The listing builds one solid part. Answer for the finished solid, in the listing's coordinates (mm). Face numbers are marked on the shaded views. A direction names the side the tool comes from. Round coordinates to 2 decimals unless told otherwise and drop trailing zeros. Write each loop counter-clockwise with the first axis right and the second up, starting at its lowest first coordinate (ties: lowest second). Pieces come first, ordered by that corner, then holes. Notation, with made-up numbers: (57, 32) - (108, 32) arc R20 cw to (108, 65) - close; hole circle Ø5 at (69.5, -26.5). An arc over 180 degrees is marked (long way). Return JSON: item names as keys, results as strings. Group by question number.
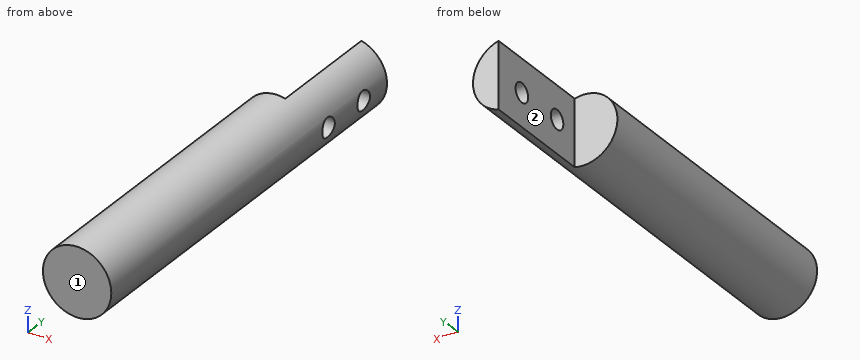
from build123d import *

# Parameters (mm, degrees)
SKETCH_1_R          = 3.175
EXTRUDE_1_DEPTH     = 57.15
CUT_EXTRUDE_1_DEPTH = 10.795
SKETCH_3_R          = 0.889
CUT_EXTRUDE_2_DEPTH = 10.795
SKETCH_4_W          = 3.926157487
SKETCH_4_H          = 0.79375
CUT_EXTRUDE_3_DEPTH = 8.573
SKETCH_5_R          = 3.774888962
CUT_EXTRUDE_4_DEPTH = 18


with BuildPart() as part:
    # 草图1 → 凸台-拉伸1 (new body)
    with BuildSketch(Plane(origin=(0, 0, 0), x_dir=(1, 0, 0), z_dir=(0, 1, 0))):
        Circle(SKETCH_1_R)
    extrude(amount=EXTRUDE_1_DEPTH)

    # 草图2 → 切除-拉伸1 (cut)
    with BuildSketch(Plane(origin=(0, 57.15, 0), x_dir=(1, 0, 0), z_dir=(0, 1, 0))):
        Polygon((-0.794, 3.175), (0.794, 3.175), (0.794, -3.175), (-3.175, -3.175), (-3.175, 3.175), align=None)
    extrude(amount=-CUT_EXTRUDE_1_DEPTH, mode=Mode.SUBTRACT)

    # 草图3 → 切除-拉伸2 (cut)
    with BuildSketch(Plane.ZY.offset(-0.794)):
        with Locations((0, 53.855)):
            Circle(SKETCH_3_R)
        with Locations((0, 48.855)):
            Circle(SKETCH_3_R)
    extrude(amount=-CUT_EXTRUDE_2_DEPTH, mode=Mode.SUBTRACT)

    # 草图4 → 切除-拉伸3 (cut)
    with BuildSketch(Plane.XZ):
        with Locations((-0.018009896, -2.778125)):
            Rectangle(SKETCH_4_W, SKETCH_4_H)
    extrude(amount=-CUT_EXTRUDE_3_DEPTH, mode=Mode.SUBTRACT)

    # 草图5 → 切除-拉伸4 (cut)
    with BuildSketch(Plane.XZ):
        Circle(SKETCH_5_R)
    extrude(amount=-CUT_EXTRUDE_4_DEPTH, mode=Mode.SUBTRACT)


solid = part.part
(1) Flat-ended cylindrical pins translate along their axes: pin 1 (1.8 mm diameter, centred on y = 50, z = -0.5, fed in from -X); pin 2 (1.5 mm diameter, centred on x = -2.5, y = 28, fed in from +Z); pin 3 (2 mm diameter, centred on x = -0.5, z = -0.5, fed in from +Y) (3 decimals); pin 4 (1.4 mm diameter, centred on y = 53.855, z = 0, fed in from +X). Find the tip coordinate at first contact, or state that the pin passes through.
(2) Find section C-C (x = 0). Write down the section's boundary in (y, z) (3 decimals), plus the area to 3 significant figures.
(3) For the marked faces 1 and 2, determine the directions among +Z, -Z, +X, -X, +Y, -Y from which every point of the face is accessible in a straight line to the end or side of a thin tool.
(4) Consider line 1 (Y direction, x = 2, z = 0); line 2 (Y direction, x = 2.75, z = 0.5); line 3 (Y direction, x = 0.25, z = 0.5) (3 decimals). Determine where each line is inside the solid, lowest interval first.
(5) Find section B-B (y = 47). Write down the section's boundary in (x, z) (3 decimals).
(6) Find section A-A (z = 0). Write down the section's boundary in (x, y) (3 decimals).
(7) Find section D-D (z = -1.75). Write down the section's boundary in (x, y) (3 decimals), plus the area to 3 significant figures.
Check sheet entries:
{
 "1": {"pin 1": "stops at x = 0.79", "pin 2": "stops at z = 2.65", "pin 3": "stops at y = 46.355", "pin 4": "passes through"},
 "2": {"outline": "(18, -3.175) - (46.355, -3.175) - (46.355, 3.175) - (18, 3.175) - close", "area": "180 mm^2"},
 "3": {"face 1": "+Z, -Z, +X, -X, -Y", "face 2": "+Z, -Z, -X, +Y"},
 "4": {"line 1": "y = 18 to 47.97, 49.74 to 52.97, 54.74 to 57.15", "line 2": "y = 18 to 48.12, 49.59 to 53.12, 54.59 to 57.15", "line 3": "y = 18 to 46.355"},
 "5": {"outline": "(0.794, -3.074) arc R3.175 ccw to (0.794, 3.074) - close"},
 "6": {"outline": "(-3.175, 18) - (3.175, 18) - (3.175, 47.966) - (0.794, 47.966) - (0.794, 46.355) - (-3.175, 46.355) - close; (0.794, 49.744) - (3.175, 49.744) - (3.175, 52.966) - (0.794, 52.966) - close; (0.794, 54.744) - (3.175, 54.744) - (3.175, 57.15) - (0.794, 57.15) - close"},
 "7": {"outline": "(-2.649, 18) - (2.649, 18) - (2.649, 57.15) - (0.794, 57.15) - (0.794, 46.355) - (-2.649, 46.355) - close", "area": "170 mm^2"}
}
